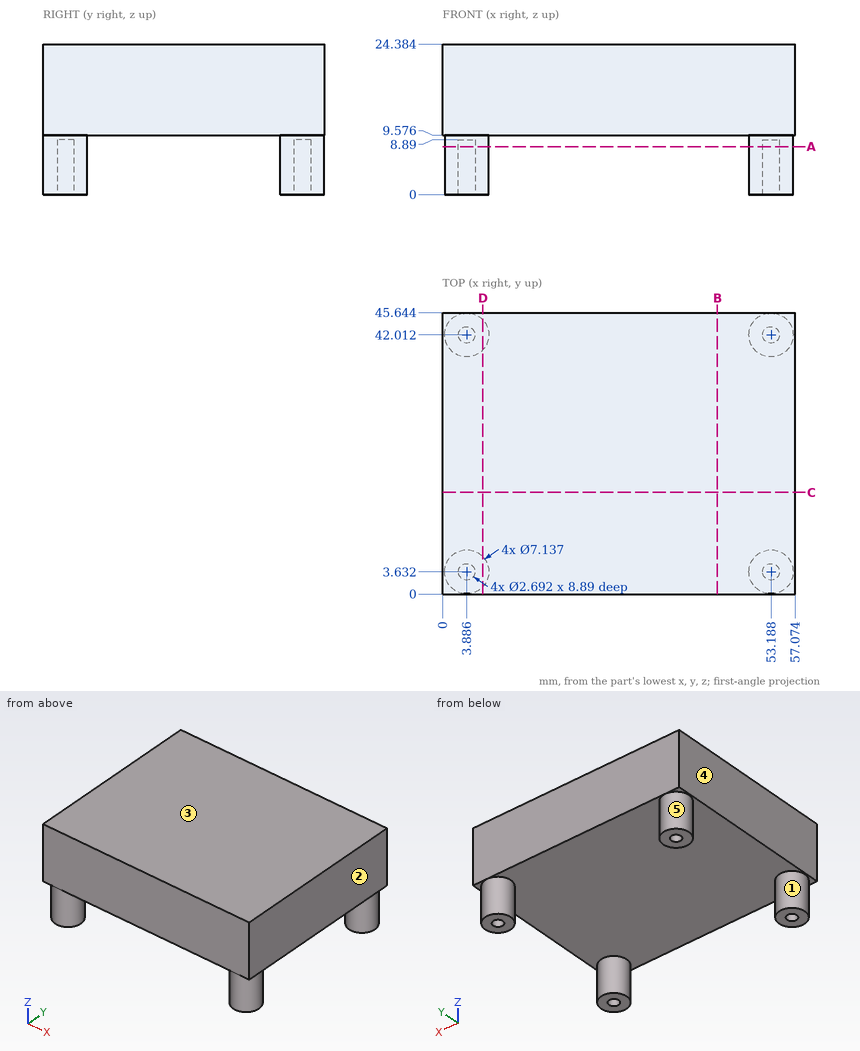
For this review, use the dimensioned drawing (mm, ordinates from the lowest corner) and the shaded views. A direction names the side the tool comes from. Coordinates: 2 decimals unless noted, no trailing zeros. Loops run counter-clockwise (first coordinate to the right, second up) from the corner with the lowest first, then second, coordinate; pieces in that order, holes last. Notation, with made-up numbers: (-21.5, -27) -> (-1.5, -27) arc R33 ccw to (-1.5, 9) -> close; hole circle Ø8 at (-13.75, 57.5). An arc over 180 degrees is marked (long way). Return JSON: item names as keys, results as strings. Group by question number.
(1) Consider section D-D, the plane x = 6.5. Give the boundary of the cut face in (y, z) (1 decimal).
(2) Consider section B-B, the plane x = 44.5. Give the boundary of the cut face in (y, z) (1 decimal).
(3) Mouldability with a two-part tool opening along X and no side actions: class the marked faces 1, 2 and 3 as pulls with the +X half, pulls with the -X half, needs draft (parallel to the pull), parting line crosses it, or undercut.
(4) Tool access review of the marked faces 4 and 5: name each direction out of +Z, -Z, +X, -X, +Y, -Y from which nothing blocks a thin tool from reaching the whole face with its end or side.
(5) Consider section A-A, the plane z = 7.75. Give the boundary of the cut face in (x, y), plus the area to 3 significant figures.
(6) For pin 1 Ø13.5 at (x, y) = (39.5, 27) entering from -Z; pin 2 Ø2 at (x, y) = (53.19, 42.01) entering from -Z, all flat-tipped, find the tip position at first contact; note any pin that passes through.
(7) To check wall thickness, follow L1, parallel to Z at x = 28.5, y = 27.5 (1 decimal); L2, parallel to X at y = 6.5, z = 1.75 (1 decimal). State the ranges of each line that lie inside material, in increasing order.
(8) Consider section C-C, the plane y = 16.5. Give the boundary of the cut face in (x, z) (1 decimal).
Results below:
{
 "1": {"outline": "(0, 9.6) -> (1.2, 9.6) -> (1.2, 0) -> (6.1, 0) -> (6.1, 9.6) -> (39.6, 9.6) -> (39.6, 0) -> (44.4, 0) -> (44.4, 9.6) -> (45.6, 9.6) -> (45.6, 24.4) -> (0, 24.4) -> close"},
 "2": {"outline": "(0, 9.6) -> (45.6, 9.6) -> (45.6, 24.4) -> (0, 24.4) -> close"},
 "3": {"face 1": "undercut", "face 2": "pulls with the +X half", "face 3": "needs draft"},
 "4": {"face 4": "+Z, -Z, -X, +Y, -Y", "face 5": "-Z"},
 "5": {"outline": "circle Ø7.14 at (3.89, 3.63); circle Ø7.14 at (3.89, 42.01); circle Ø7.14 at (53.19, 3.63); circle Ø7.14 at (53.19, 42.01); hole circle Ø2.69 at (3.89, 3.63); hole circle Ø2.69 at (3.89, 42.01); hole circle Ø2.69 at (53.19, 3.63); hole circle Ø2.69 at (53.19, 42.01)", "area": "137 mm2"},
 "6": {"pin 1": "stops at z = 9.58", "pin 2": "stops at z = 8.89"},
 "7": {"L1": "z = 9.6 to 24.4", "L2": "x = 1.8 to 6, 51.1 to 55.3"},
 "8": {"outline": "(0, 9.6) -> (57.1, 9.6) -> (57.1, 24.4) -> (0, 24.4) -> close"}
}
